Check sheet for the modelled part. Datum: model origin and axes. Units: mm. Round coordinates to 2 decimals unless told otherwise and drop trailing zeros. Loops run counter-clockwise (first coordinate to the right, second up) from the corner with the lowest first, then second, coordinate; pieces in that order, holes last. Notation, with made-up numbers: (39, 75) -> (51, 75) arc R25 cw to (51, 89) -> close; hole circle Ø6 at (51.5, -16.5). An arc over 180 degrees is marked (long way). Use one line per item in the form item = value. Start each with the question number.
(1) Sectioned sample at B-B (z = -32). Record the cut outline in (x, y), and give its area (3 significant figures).
(2) Sectioned sample at C-C (z = -53.5). Record the cut outline in (x, y).
(3) Go/stop test with flat-tipped pins: pin 1 (1.2 mm diameter, centred on x = 2.5, z = -65, fed in from -Y); pin 2 (1.2 mm diameter, centred on x = 1.5, z = -65, fed in from +Y); pin 3 (1.5 mm diameter, centred on x = 1.5, z = 39, fed in from -Y); pin 4 (6 mm diameter, centred on y = 2.5, z = -48.5, fed in from -X). Record where each tip stops, or that it passes through.
(4) Sectioned sample at A-A (x = 3.1). Record the cut outline in (y, z), and give its area (4 significant figures).
(5) Material ranges on probe 1 along Y at (x, z) = (0.8, 60); probe 2 along Y at (x, z) = (2.2, 42), recorded low to high. Write a range as [from, to].
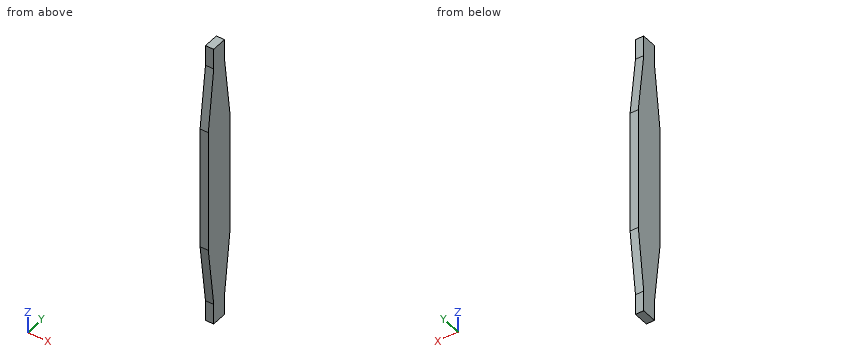
from build123d import *

# Parameters (mm, degrees)
SKETCH_1_W      = 60
SKETCH_1_H      = 15
SKETCH_1_W_2    = 10
SKETCH_1_H_2    = 7.5
EXTRUDE_1_DEPTH = 4


with BuildPart() as part:
    # Эскиз1 → Бобышка-Вытянуть1 (new body)
    with BuildSketch(Plane(origin=(0, 0, 0), x_dir=(0, 0, -1), z_dir=(1, 0, 0))):
        Rectangle(SKETCH_1_W, SKETCH_1_H)
        Polygon((-30, -7.5), (-30, 7.5), (-60, 3.75), (-60, -3.75), align=None)
        with Locations((-65, 0)):
            Rectangle(SKETCH_1_W_2, SKETCH_1_H_2)
        Polygon((60, -3.75), (30, -7.5), (30, 7.5), (60, 3.75), align=None)
        with Locations((65, 0)):
            Rectangle(SKETCH_1_W_2, SKETCH_1_H_2)
    extrude(amount=EXTRUDE_1_DEPTH)


solid = part.part
Checks:
q1.outline = (0, -7.25) -> (4, -7.25) -> (4, 7.25) -> (0, 7.25) -> close
q1.area = 58.0 mm2
q2.outline = (0, -4.56) -> (4, -4.56) -> (4, 4.56) -> (0, 4.56) -> close
q3.pin_1 = -3.75
q3.pin_2 = 3.75
q3.pin_3 = -6.47
q3.pin_4 = 0
q4.outline = (-7.5, -30) -> (-3.75, -60) -> (-3.75, -70) -> (3.75, -70) -> (3.75, -60) -> (7.5, -30) -> (7.5, 30) -> (3.75, 60) -> (3.75, 70) -> (-3.75, 70) -> (-3.75, 60) -> (-7.5, 30) -> close
q4.area = 1,725 mm2
q5.probe_1 = [-3.75, 3.75]
q5.probe_2 = [-6, 6]
